Part model, mm, in its own coordinate system. A direction names the side the tool comes from. Round coordinates to 2 decimals unless told otherwise and drop trailing zeros. Write each loop counter-clockwise with the first axis right and the second up, starting at its lowest first coordinate (ties: lowest second). Pieces come first, ordered by that corner, then holes. Notation, with made-up numbers: (-18.75, 11.5) -> (-7.75, 11.5) arc R26 cw to (-7.75, 32.5) -> close; hole circle Ø4 at (28.5, 69). An arc over 180 degrees is marked (long way). Return JSON: item names as keys, results as strings. Group by question number.
(1) Drop flat-ended pins along their axis: pin 1 Ø3 at (y, z) = (14.5, -25.11) entering from +X; pin 2 Ø3.5 at (y, z) = (-0.5, 2) entering from +X; pin 3 Ø4 at (x, z) = (-8.5, -8.5) entering from +Y; pin 4 Ø5 at (x, y) = (-6.5, 17.5) entering from +Z. Give the stop position or say it passes through.
(2) Mould opens along Y. For faces 1 (the flat face through (-8, 0, 0)), 2 (the flat face through (0, 0, -7)), 3 (the cylindrical face through (-2.958, 34.168, 7.587)) say: +Y half, -Y half, draft (parallel to the pull), parting line (faces both ways), or undercut.
(3) Tool access for faces 4 (the cylindrical face through (-3.94, -5.37, 1.19)), 5 (the cylindrical face through (-3.55, 31.48, -0.33)), 6 (the flat face through (-7, 17.5, -17.5)): list every direction of +Z, -Z, +X, -X, +Y, -Y with a clear straight run to the whole face (end or side of a thin tool).
(4) Saw through at B-B (y = 0). List the corners of the cut face in (x, z), plus the area to 3 significant figures.
(5) Drill centre lines: L1, parallel to Y at x = -1.25, z = 0; L2, parallel to Y at x = -6, z = -25; L3, parallel to X at y = 18.5, z = 21.5. Where is each one in solid material? Low to high. Write a range as from..to.
(6) Saw through at D-D (y = 13.5). State how many separate pieces and enclosed holes the cut face has, plus the area to 3 significant figures.
(7) Saw through at C-C (x = -2). List the corners of the cut face in (y, z).
(8) Saw through at A-A (z = 0). List the corners of the cut face in (x, y), plus the area to 3 significant figures.
from build123d import *

# Parameters (mm, degrees)
SCHIZZO1_W               = 7
SCHIZZO1_H               = 35
SCHIZZO2_R               = 2.5
TAGLIO_ESTRUSIONE1_DEPTH = 50.989999
SCHIZZO3_R               = 5.5
TAGLIO_ESTRUSIONE2_DEPTH = 8
RACCORDO1_R              = 1
SMUSSO1_SIZE             = 1


with BuildPart() as part:
    # Schizzo1 → Rivoluzione1 (revolve)
    with BuildSketch(Plane(origin=(0, 0, 0), x_dir=(1, 0, 0), z_dir=(0, 1, 0)), mode=Mode.PRIVATE) as rivoluzione1_sk:
        Polygon((-7, -24), (-7, 0), (-12, 0), (-12, -10), align=None)
        with Locations((-3.5, -17.5)):
            Rectangle(SCHIZZO1_W, SCHIZZO1_H)
    revolve(rivoluzione1_sk.sketch.rotate(Axis((0, 0, 0), (-1, 0, 0)), 180), axis=Axis((0, 0, 0), (-1, 0, 0)))

    # Schizzo2 → Taglio-Estrusione1 (cut, through all)
    with BuildSketch(Plane.ZY.offset(7)):
        with Locations((0, 29)):
            Circle(SCHIZZO2_R)
        with Locations((-25.11473671, 14.5)):
            Circle(SCHIZZO2_R)
        with Locations((-25.11473671, -14.5)):
            Circle(SCHIZZO2_R)
        with Locations((0, -29)):
            Circle(SCHIZZO2_R)
        with Locations((25.11473671, -14.5)):
            Circle(SCHIZZO2_R)
        with Locations((25.11473671, 14.5)):
            Circle(SCHIZZO2_R)
    extrude(amount=-TAGLIO_ESTRUSIONE1_DEPTH, mode=Mode.SUBTRACT)

    # Schizzo3 → Taglio-Estrusione2 (cut)
    with BuildSketch(Plane(origin=(0, 0, 0), x_dir=(0, 0, -1), z_dir=(1, 0, 0))):
        Circle(SCHIZZO3_R)
    extrude(amount=-TAGLIO_ESTRUSIONE2_DEPTH, mode=Mode.SUBTRACT)

    # Raccordo1
    raccordo1_edges = [part.edges().sort_by_distance(p)[0] for p in [
        (-7, 0, 24),
    ]]
    fillet(raccordo1_edges, radius=RACCORDO1_R)

    # Smusso1
    smusso1_edges = [part.edges().sort_by_distance(p)[0] for p in [
        (-7, 0, 35),
    ]]
    chamfer(smusso1_edges, length=SMUSSO1_SIZE)


solid = part.part
Computed values:
{
 "1": {"pin 1": "through", "pin 2": "x = -8", "pin 3": "y = 33.49", "pin 4": "z = 31.6"},
 "2": {"face 1": "undercut", "face 2": "draft", "face 3": "parting line"},
 "3": {"face 4": "+X", "face 5": "+X, -X", "face 6": "-X"},
 "4": {"outline": "(-12, -10) -> (-7.06, -23.84) arc R1 cw to (-7, -24.17) -> (-7, -34) -> (-6, -35) -> (0, -35) -> (0, -5.5) -> (-8, -5.5) -> (-8, 5.5) -> (0, 5.5) -> (0, 35) -> (-6, 35) -> (-7, 34) -> (-7, 24.17) arc R1 cw to (-7.06, 23.84) -> (-12, 10) -> close", "area": "571 mm2"},
 "5": {"L1": "-35..-31.5, -26.5..-5.5, 5.5..26.5, 31.5..35", "L2": "-24.49..-17, -12..12, 17..24.49", "L3": "-7..0"},
 "6": {"separate pieces": "3", "enclosed holes": "0", "area": "480 mm2"},
 "7": {"outline": "circle Ø70 at (0, 0); hole circle Ø5 at (-29, 0); hole circle Ø5 at (-14.5, -25.11); hole circle Ø5 at (-14.5, 25.11); hole circle Ø11 at (0, 0); hole circle Ø5 at (14.5, -25.11); hole circle Ø5 at (14.5, 25.11); hole circle Ø5 at (29, 0)"},
 "8": {"outline": "(-12, -10) -> (-7.06, -23.84) arc R1 cw to (-7, -24.17) -> (-7, -26.5) -> (0, -26.5) -> (0, -5.5) -> (-8, -5.5) -> (-8, 5.5) -> (0, 5.5) -> (0, 26.5) -> (-7, 26.5) -> (-7, 24.17) arc R1 cw to (-7.06, 23.84) -> (-12, 10) -> close; (-7, -34) -> (-6, -35) -> (0, -35) -> (0, -31.5) -> (-7, -31.5) -> close; (-7, 31.5) -> (0, 31.5) -> (0, 35) -> (-6, 35) -> (-7, 34) -> close", "area": "501 mm2"}
}
